Can you work these out from the model? Positions are in its coordinate system, mm. Give positions to 0.01 mm unless a question says otherwise; leave off trailing zeros. Loops run counter-clockwise (first coordinate to the right, second up) from the corner with the lowest first, then second, coordinate; pieces in that order, holes last. Notation, with made-up numbers: M -12,87.25 L -1,87.25 A27 cw -1,112.25 Z; hole C 50,7 d5. An arc over 180 degrees is marked long. One line per item, written item: value. Start each with the question number.
from build123d import *

# Parameters (mm, degrees)
SKETCH1_W                       = 31.4
SKETCH1_H                       = 31.4
SKETCH1_R                       = 10.25
BOSS_EXTRUDE1_DEPTH             = 40
SKETCH2_R                       = 1.5
CUT_EXTRUDE1_DEPTH              = 40
M4_TAPPED_HOLE1_D               = 3.3
M4_TAPPED_HOLE1_DEPTH           = 10.1
M4_TAPPED_HOLE1_TIP             = 0.991420021
M4_TAPPED_HOLE1_ON_FACE_2_D     = 3.3
M4_TAPPED_HOLE1_ON_FACE_2_DEPTH = 10.1
M4_TAPPED_HOLE1_ON_FACE_2_TIP   = 0.991420021
SKETCH5_R                       = 1.5
CUT_EXTRUDE2_DEPTH              = 40
M4_TAPPED_HOLE2_D               = 3.3
M4_TAPPED_HOLE2_DEPTH           = 10.1
M4_TAPPED_HOLE2_TIP             = 0.991420021
M4_TAPPED_HOLE2_ON_FACE_2_D     = 3.3
M4_TAPPED_HOLE2_ON_FACE_2_DEPTH = 10.1
M4_TAPPED_HOLE2_ON_FACE_2_TIP   = 0.991420021
SKETCH8_R                       = 1.5
CUT_EXTRUDE3_DEPTH              = 30
M4_TAPPED_HOLE3_D               = 3.3
M4_TAPPED_HOLE3_DEPTH           = 52.1
M4_TAPPED_HOLE3_TIP             = 0.991420021


with BuildPart() as part:
    # Sketch1 → Boss-Extrude1 (new body)
    with BuildSketch(Plane(origin=(0, 0, 0), x_dir=(1, 0, 0), z_dir=(0, 1, 0))):
        Rectangle(SKETCH1_W, SKETCH1_H)
        with Locations(Location((0, 0, 0), (0, 0, 270))):
            Circle(SKETCH1_R, mode=Mode.SUBTRACT)
    extrude(amount=BOSS_EXTRUDE1_DEPTH)

    # Sketch2 → Cut-Extrude1 (cut)
    with BuildSketch(Plane(origin=(15.7, 0, 0), x_dir=(0, 0, -1), z_dir=(1, 0, 0))):
        with Locations((0, 30)):
            Circle(SKETCH2_R)
        with Locations((0, 10)):
            Circle(SKETCH2_R)
    extrude(amount=-CUT_EXTRUDE1_DEPTH, mode=Mode.SUBTRACT)

    # M4 Tapped Hole1
    with Locations(Plane(origin=(-15.7, 10, 0), x_dir=(0, 0, -1), z_dir=(-1, 0, 0))):
        with Locations((0, 0), (0, -20)):
            Hole(M4_TAPPED_HOLE1_D / 2, depth=M4_TAPPED_HOLE1_DEPTH)
            with Locations((0, 0, -(M4_TAPPED_HOLE1_DEPTH + M4_TAPPED_HOLE1_TIP / 2))):  # 118° drill point
                Cone(0, M4_TAPPED_HOLE1_D / 2, M4_TAPPED_HOLE1_TIP, mode=Mode.SUBTRACT)

    # M4 Tapped Hole1 on face 2
    with Locations(Plane(origin=(15.7, 30, 0), x_dir=(0, 0, -1), z_dir=(-1, 0, 0))):
        with Locations((0, 0), (0, 20)):
            Hole(M4_TAPPED_HOLE1_ON_FACE_2_D / 2, depth=M4_TAPPED_HOLE1_ON_FACE_2_DEPTH)
            with Locations((0, 0, -(M4_TAPPED_HOLE1_ON_FACE_2_DEPTH + M4_TAPPED_HOLE1_ON_FACE_2_TIP / 2))):  # 118° drill point
                Cone(0, M4_TAPPED_HOLE1_ON_FACE_2_D / 2, M4_TAPPED_HOLE1_ON_FACE_2_TIP, mode=Mode.SUBTRACT)

    # Sketch5 → Cut-Extrude2 (cut)
    with BuildSketch(Plane.XY.offset(15.7)):
        with Locations((0, 30)):
            Circle(SKETCH5_R)
        with Locations((0, 10)):
            Circle(SKETCH5_R)
    extrude(amount=-CUT_EXTRUDE2_DEPTH, mode=Mode.SUBTRACT)

    # M4 Tapped Hole2
    with Locations(Plane(origin=(0, 30, 15.7), x_dir=(1, 0, 0), z_dir=(0, 0, 1))):
        with Locations((0, 0), (0, -20)):
            Hole(M4_TAPPED_HOLE2_D / 2, depth=M4_TAPPED_HOLE2_DEPTH)
            with Locations((0, 0, -(M4_TAPPED_HOLE2_DEPTH + M4_TAPPED_HOLE2_TIP / 2))):  # 118° drill point
                Cone(0, M4_TAPPED_HOLE2_D / 2, M4_TAPPED_HOLE2_TIP, mode=Mode.SUBTRACT)

    # M4 Tapped Hole2 on face 2
    with Locations(Plane(origin=(0, 30, -15.7), x_dir=(1, 0, 0), z_dir=(0, 0, 1))):
        with Locations((0, 0), (0, -20)):
            Hole(M4_TAPPED_HOLE2_ON_FACE_2_D / 2, depth=M4_TAPPED_HOLE2_ON_FACE_2_DEPTH)
            with Locations((0, 0, -(M4_TAPPED_HOLE2_ON_FACE_2_DEPTH + M4_TAPPED_HOLE2_ON_FACE_2_TIP / 2))):  # 118° drill point
                Cone(0, M4_TAPPED_HOLE2_ON_FACE_2_D / 2, M4_TAPPED_HOLE2_ON_FACE_2_TIP, mode=Mode.SUBTRACT)

    # Sketch8 → Cut-Extrude3 (cut)
    with BuildSketch(Plane.XZ):
        with Locations(Location((-10.7, 10.7, 0), (0, 0, 270))):
            Circle(SKETCH8_R)
        with Locations(Location((10.7, 10.7, 0), (0, 0, 90))):
            Circle(SKETCH8_R)
        with Locations(Location((10.7, -10.7, 0), (0, 0, 270))):
            Circle(SKETCH8_R)
        with Locations(Location((-10.7, -10.7, 0), (0, 0, 90))):
            Circle(SKETCH8_R)
    extrude(amount=-CUT_EXTRUDE3_DEPTH, mode=Mode.SUBTRACT)

    # M4 Tapped Hole3
    with Locations(Plane(origin=(-10.7, 0, 10.7), x_dir=(0, 0, -1), z_dir=(0, -1, 0))):
        with Locations((0, 0), (0, 21.4), (21.4, 21.4), (21.4, 0)):
            Hole(M4_TAPPED_HOLE3_D / 2, depth=M4_TAPPED_HOLE3_DEPTH)
            with Locations((0, 0, -(M4_TAPPED_HOLE3_DEPTH + M4_TAPPED_HOLE3_TIP / 2))):  # 118° drill point
                Cone(0, M4_TAPPED_HOLE3_D / 2, M4_TAPPED_HOLE3_TIP, mode=Mode.SUBTRACT)


solid = part.part
Q1. If we mould it in two halves opening along Z, with no side actions, what happens to faces 1 (the face through (0.215, 31.636, 12.869)), 2 (the face through (12.9, 11.6, -0.4)), 3 (the face through (0, 20, -15.7)), 4 (the face through (0, 20, 15.7))? For each: released by +Z, released by -Z, zero draft, split by the parting line, or undercut.
Q2. If we section it at A-A, the plane x = 0: Write out the boundary of the cut face in (y, z), plus the area to 3 significant figures.
Q3. If we section it at B-B, the plane y = 37: Write out the boundary of the cut face in (x, z).
Q4. If we section it at C-C, the plane z = 11: Write out the boundary of the cut face in (x, y), plus the area to 3 significant figures.
Q5. If we section it at D-D, the plane y = 31: Write out the boundary of the cut face in (x, z).
Q6. I need wall thicknesses on line 1 along Y through (x, z) = (0, -14.5); line 2 along Z through (x, y) = (-14.25, 30); line 3 along X through (y, z) = (18.5, 10.7). Which ranges of each line are inside material? Lowest first, please.
Response:
1. face 1: zero draft
1. face 2: undercut
1. face 3: released by -Z
1. face 4: released by +Z
2. outline: M 0,-15.7 L 8.35,-15.7 L 8.35,-10.25 L 0,-10.25 Z; M 0,10.25 L 8.35,10.25 L 8.35,15.7 L 0,15.7 Z; M 11.65,-15.7 L 28.35,-15.7 L 28.35,-10.25 L 11.65,-10.25 Z; M 11.65,10.25 L 28.35,10.25 L 28.35,15.7 L 11.65,15.7 Z; M 31.65,-15.7 L 40,-15.7 L 40,-10.25 L 31.65,-10.25 Z; M 31.65,10.25 L 40,10.25 L 40,15.7 L 31.65,15.7 Z
2. area: 364 mm^2
3. outline: M -15.7,-15.7 L 15.7,-15.7 L 15.7,15.7 L -15.7,15.7 Z; hole C -10.7,-10.7 d3.3; hole C -10.7,10.7 d3.3; hole C 0,0 d20.5; hole C 10.7,-10.7 d3.3; hole C 10.7,10.7 d3.3
4. outline: M -15.7,0 L -12.32,0 L -12.32,40 L -15.7,40 Z; M -9.08,0 L 9.08,0 L 9.08,40 L -9.08,40 Z; M 12.32,0 L 15.7,0 L 15.7,40 L 12.32,40 Z; hole C 0,10 d3.3; hole C 0,30 d3.3
4. area: 979 mm^2
5. outline: M -15.7,-15.7 L -1.31,-15.7 L -1.31,-10.17 A10.25 cw -10.17,-1.31 L -15.7,-1.31 Z; M -15.7,1.31 L -10.17,1.31 A10.25 cw -1.31,10.17 L -1.31,15.7 L -15.7,15.7 Z; M 1.31,-15.7 L 15.7,-15.7 L 15.7,-1.31 L 10.17,-1.31 A10.25 cw 1.31,-10.17 Z; M 1.31,10.17 A10.25 cw 10.17,1.31 L 15.7,1.31 L 15.7,15.7 L 1.31,15.7 Z; hole C -10.7,-10.7 d3.3; hole C -10.7,10.7 d3.3; hole C 10.7,-10.7 d3.3; hole C 10.7,10.7 d3.3
6. line 1: 0 to 8.35, 11.65 to 28.35, 31.65 to 40
6. line 2: -15.7 to -1.65, 1.65 to 15.7
6. line 3: -15.7 to -12.35, -9.05 to 9.05, 12.35 to 15.7
